Verification items for the finished model (mm, model axes). Face numbers are marked on the shaded views. A direction names the side the tool comes from. Round coordinates to 2 decimals unless told otherwise and drop trailing zeros. Write each loop counter-clockwise with the first axis right and the second up, starting at its lowest first coordinate (ties: lowest second). Pieces come first, ordered by that corner, then holes. Notation, with made-up numbers: (-9, -25.75) - (0, -25.75) arc R14 cw to (0, -11.75) - close; hole circle Ø11 at (-5, -28). An arc over 180 degrees is marked (long way). Answer as a JSON object with one key per item and string values.
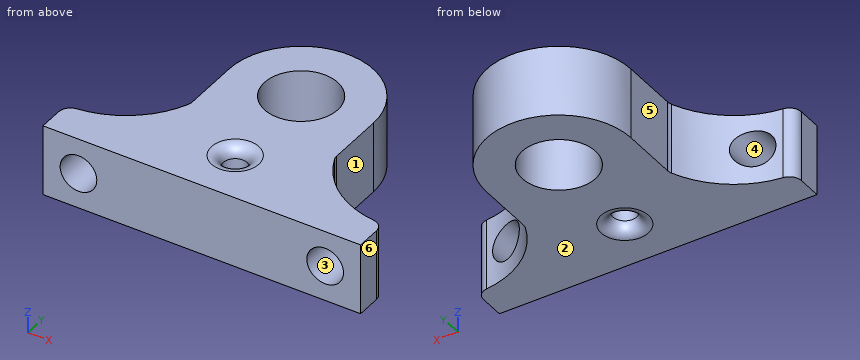
```python
from build123d import *

# Parameters (mm, degrees)
SKETCH1_R               = 3.1
SKETCH1_R_2             = 1
BOSS_EXTRUDE1_DEPTH     = 6
CUT_EXTRUDE1_DEPTH      = 25.107196906
CUT_EXTRUDE1_DEPTH_BACK = 25.107196906
SKETCH2_R               = 1.55
FILLET1_R               = 1


with BuildPart() as part:
    # Sketch1 → Boss-Extrude1 (new body)
    with BuildSketch(Plane.XY):
        with BuildLine():
            Line((-6.1, 0), (-6.1, -4.807578818))
            ThreePointArc((-6.1, -4.807578818), (-6.119327431, -5.003234924), (-6.176562624, -5.191327971))
            ThreePointArc((-6.176562624, -5.191327971), (-9.070412736, -8.700522421), (-13.42933143, -10))
            Line((-13.42933143, -10), (-13.42933143, -13))
            Line((-13.42933143, -13), (13.42933143, -13))
            Line((13.42933143, -13), (13.42933143, -10))
            ThreePointArc((13.42933143, -10), (9.070412736, -8.700522421), (6.176562624, -5.191327971))
            ThreePointArc((6.176562624, -5.191327971), (6.119327431, -5.003234924), (6.1, -4.807578818))
            Line((6.1, -4.807578818), (6.1, 0))
            ThreePointArc((6.1, 0), (0, 6.1), (-6.1, 0))
        make_face()
        Circle(SKETCH1_R, mode=Mode.SUBTRACT)
        with Locations((0, -8.629378488)):
            Circle(SKETCH1_R_2, mode=Mode.SUBTRACT)
    extrude(amount=BOSS_EXTRUDE1_DEPTH)

    # Sketch2 → Cut-Extrude1 (cut, two sides: drawn at the far end of the back side and taken through both)
    with BuildSketch(Plane.XZ.offset(13).offset(-CUT_EXTRUDE1_DEPTH_BACK)):
        with Locations((-10.42933143, 3)):
            Circle(SKETCH2_R)
        with Locations((10.42933143, 3)):
            Circle(SKETCH2_R)
    extrude(amount=CUT_EXTRUDE1_DEPTH + CUT_EXTRUDE1_DEPTH_BACK, mode=Mode.SUBTRACT)

    # Fillet1
    fillet1_edges = [part.edges().sort_by_distance(p)[0] for p in [
        (-1, -8.629378488, 0),
        (13.42933143, -10, 3),
        (-13.42933143, -10, 3),
        (-1, -8.629378488, 6),
    ]]
    fillet(fillet1_edges, radius=FILLET1_R)


solid = part.part
```
Q1. Section check C-C, the plane y = -2. Record the cut outline in (x, z).
Geometry check:
{"outline": "(-6.1, 0) - (-2.37, 0) - (-2.37, 6) - (-6.1, 6) - close; (2.37, 0) - (6.1, 0) - (6.1, 6) - (2.37, 6) - close"}
Q2. Gauge pin test, flat ends, axial feed: P1, Ø3, axis at x = 10.43, z = 3, coming from the +Y side; P2, Ø1.4, axis at y = -3.5, z = 4.5, coming from the +X side; P3, Ø10, axis at x = 0, y = 0, coming from the -Z side; P4, Ø3, axis at y = 1, z = 3.5, coming from the -X side. Record the tip position at first contact, or that the pin passes through.
Geometry check:
{"P1": "passes through", "P2": "stops at x = 6.1", "P3": "stops at z = 0", "P4": "stops at x = -6.1"}
Q3. Section check A-A, the plane x = 0. Record the cut outline in (y, z).
Geometry check:
{"outline": "(-13, 0) - (-10.63, 0) arc R1 ccw to (-9.63, 1) - (-9.63, 5) arc R1 ccw to (-10.63, 6) - (-13, 6) - close; (-7.63, 1) arc R1 ccw to (-6.63, 0) - (-3.1, 0) - (-3.1, 6) - (-6.63, 6) arc R1 ccw to (-7.63, 5) - close; (3.1, 0) - (6.1, 0) - (6.1, 6) - (3.1, 6) - close"}
Q4. Section check D-D, the plane x = -9.75. Record the cut outline in (y, z), then the cut area to 3 significant figures.
Geometry check:
{"outline": "(-13, 0) - (-9.1, 0) - (-9.1, 1.61) - (-13, 1.61) - close; (-13, 4.39) - (-9.1, 4.39) - (-9.1, 6) - (-13, 6) - close", "area": "12.5 mm2"}
Q5. Release check for a two-part mould opening along Z. For the marked faces 1, 2, 3 and 4 record: released by +Z, released by -Z, zero draft, split by the parting line, or undercut.
Geometry check:
{"face 1": "zero draft", "face 2": "released by -Z", "face 3": "undercut", "face 4": "undercut"}
Q6. Set-up check for the marked faces 5 and 6: record each of +Z, -Z, +X, -X, +Y, -Y from which the full face is reachable in a straight line by a thin tool's end or side.
Geometry check:
{"face 5": "+Z, -Z, -X, +Y", "face 6": "+Z, -Z, +X, +Y, -Y"}
Q7. Material ranges on line 1 along X through (y, z) = (-10.9, 3); line 2 along Y through (x, z) = (0, 1.85); line 3 along X through (y, z) = (-10.4, 3), recorded low to high. Write a range as [from, to].
Geometry check:
{"line 1": "x = [-13.43, -11.98], [-8.88, 8.88], [11.98, 13.43]", "line 2": "y = [-13, -9.63], [-7.63, -3.1], [3.1, 6.1]", "line 3": "x = [-13.27, -11.98], [-8.88, 8.88], [11.98, 13.27]"}
Q8. Section check B-B, the plane z = 3. Record the cut outline in (x, y), then the cut area to 3 significant figures.
Geometry check:
{"outline": "(-13.43, -13) - (-11.98, -13) - (-11.98, -9.87) arc R7.8 cw to (-12.54, -9.95) arc R1 ccw to (-13.43, -10.95) - close; (-8.88, -13) - (8.88, -13) - (8.88, -8.57) arc R7.8 cw to (6.18, -5.19) arc R1 cw to (6.1, -4.81) - (6.1, 0) arc R6.1 ccw to (-6.1, 0) - (-6.1, -4.81) arc R1 cw to (-6.18, -5.19) arc R7.8 cw to (-8.88, -8.57) - close; (11.98, -13) - (13.43, -13) - (13.43, -10.95) arc R1 ccw to (12.54, -9.95) arc R7.8 cw to (11.98, -9.87) - close; hole circle Ø6.2 at (0, 0); hole circle Ø2 at (0, -8.63)", "area": "225 mm2"}
